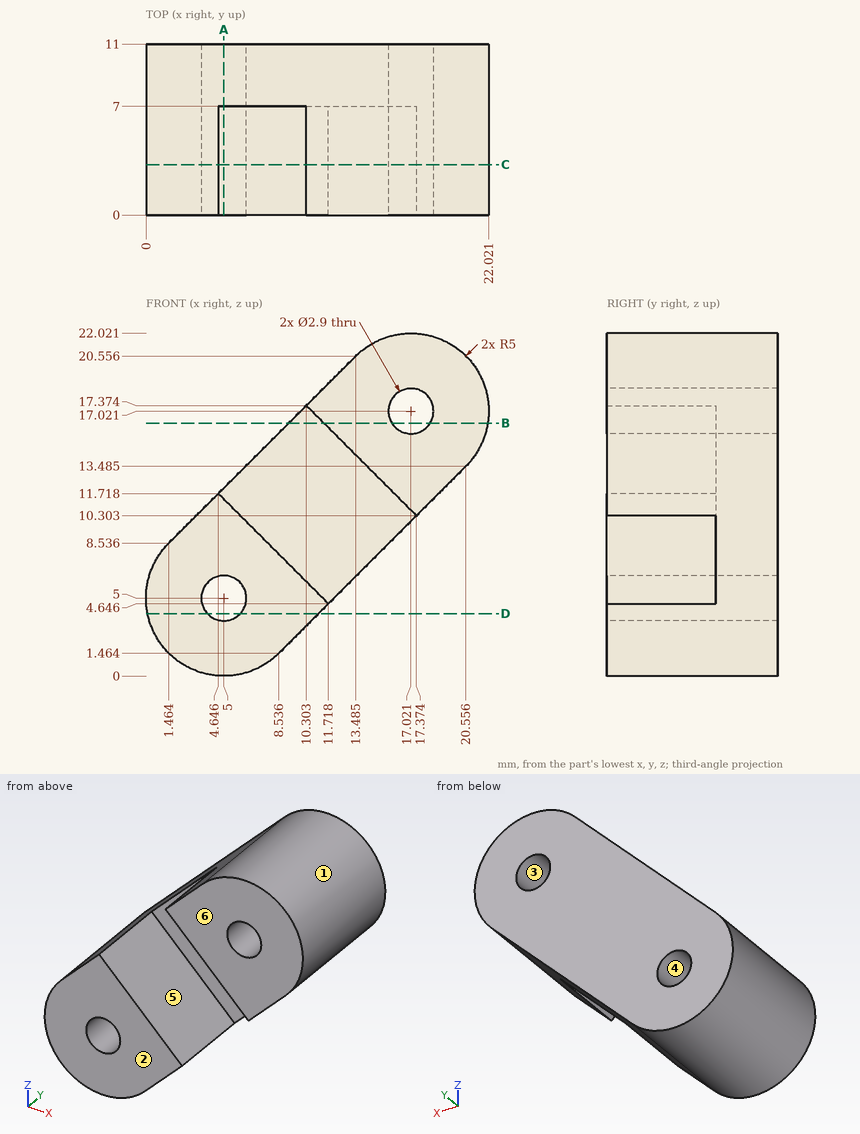
Can you work these out from the drawing? Everything is in mm from the part's minimum corner. A direction names the side the tool comes from. Give positions to 0.01 mm unless a question says otherwise; leave off trailing zeros. Write each loop counter-clockwise with the first axis right and the second up, starting at its lowest first coordinate (ties: lowest second). Pieces come first, ordered by that corner, then holes. Notation, with made-up numbers: M -6,1 L 8,1 A33 cw 8,37 Z; hole C 44,27.25 d6. An arc over 180 degrees is marked long. Answer in a Markdown table with one row per item. Add a question column.
Item 1: For pin 1 Ø3 at (x, z) = (4.5, 13.5) entering from -Y; pin 2 Ø6 at (y, z) = (2, 10) entering from +X; pin 3 Ø2 at (y, z) = (3, 2.5) entering from -X; pin 4 Ø3.5 at (x, z) = (5, 5) entering from -Y, each with a flat end and sliding along its axis, tell me the tip position at first contact or that it passes through.
Item 2: Please list where these lines run through material, in increasing order: L1, parallel to Y at x = 13, z = 6.25; L2, parallel to Z at x = 19, y = 5 (1 decimal); L3, parallel to Z at x = 11.5, y = 9.
Item 3: Imagine slicing it at C-C, the plane y = 3.25. State how many separate pieces and enclosed holes the cut face has, plus the area to 3 significant figures.
Item 4: Imagine slicing it at B-B, the plane z = 16.25. Write out the boundary of the cut face in (x, y).
Item 5: On a 3-axis mill with a long thin cutter (end or side, diameter ignored), from which of +Z, -Z, +X, -X, +Y, -Y can I reach the whole of each face in a straight line? I mean the marked faces 5 and 6. Say none if no direction works.
Item 6: Imagine slicing it at D-D, the plane z = 4. Write out the boundary of the cut face in (x, y).
Item 7: We'd pull the mould along Z, two halves only. Please class the marked faces 1, 2, 3 and 4: released by +Z, released by -Z, zero draft, split by the parting line, or undercut.
Item 8: Imagine slicing it at A-A, the plane x = 5. Write out the boundary of the cut face in (y, z).
Evaluation:
| question | item | result |
|---|---|---|
| 1 | pin 1 | stops at y = 7 |
| 1 | pin 2 | stops at x = 20.07 |
| 1 | pin 3 | stops at x = 0.23 |
| 1 | pin 4 | stops at y = 0 |
| 2 | L1 | y = 7 to 11 |
| 2 | L2 | z = 11.9 to 21.6 |
| 2 | L3 | z = 4.43 to 18.57 |
| 3 | separate pieces | 2 |
| 3 | enclosed holes | 2 |
| 3 | area | 155 mm² |
| 4 | outline | M 9.18,7 L 11.43,7 L 11.43,0 L 15.79,0 L 15.79,11 L 9.18,11 Z; M 18.25,0 L 21.96,0 L 21.96,11 L 18.25,11 Z |
| 5 | face 5 | -Y |
| 5 | face 6 | +Z, -Z, +X, -X, -Y |
| 6 | outline | M 0.1,0 L 3.95,0 L 3.95,11 L 0.1,11 Z; M 6.05,0 L 11.07,0 L 11.07,11 L 6.05,11 Z |
| 7 | face 1 | split by the parting line |
| 7 | face 2 | zero draft |
| 7 | face 3 | undercut |
| 7 | face 4 | undercut |
| 8 | outline | M 0,0 L 11,0 L 11,3.55 L 0,3.55 Z; M 0,6.45 L 11,6.45 L 11,12.07 L 7,12.07 L 7,11.36 L 0,11.36 Z |
